Work out the finished part from the listing and answer in its coordinate system (mm). Face numbers are marked on the shaded views. A direction names the side the tool comes from. Give positions to 0.01 mm unless a question says otherwise; leave off trailing zeros. Loops run counter-clockwise (first coordinate to the right, second up) from the corner with the lowest first, then second, coordinate; pieces in that order, holes last.
```python
from build123d import *

# Parameters (mm, degrees)
EXTRUDE_1_DEPTH     = 18
HOLE_WIZARD_M6_1_D  = 5
SKETCH_6_R          = 3
CUT_EXTRUDE_1_DEPTH = 259.015029546
SKETCH_7_R          = 11
SKETCH_7_R_2        = 1.25
CUT_EXTRUDE_2_DEPTH = 259.015029546


with BuildPart() as part:
    # 草图1 → 凸台-拉伸1 (new body)
    with BuildSketch(Plane.XY):
        Polygon((0, 0), (80, 0), (80, 60), (22.986425339, 129.63800905), (22.986425339, 244.63800905), (-47.013574661, 244.63800905), (-47.013574661, 104.63800905), (0, 47.214285714), align=None)
    extrude(amount=EXTRUDE_1_DEPTH)

    # M6 螺纹孔1 (through all)
    with Locations(Plane.XY.offset(18)):
        with Locations((-40.013574661, 114.63800905), (-22.013574661, 114.63800905), (-40.013574661, 234.63800905), (-22.013574661, 234.63800905), (-42.013574661, 174.63800905)):
            Hole(HOLE_WIZARD_M6_1_D / 2)

    # 草图6 → 切除-拉伸1 (cut, through all)
    with BuildSketch(Plane.XY.offset(18)):
        with Locations((15, 20)):
            Circle(SKETCH_6_R)
        with Locations((65, 20)):
            Circle(SKETCH_6_R)
        with Locations((40, 20)):
            Circle(SKETCH_6_R)
    extrude(amount=-CUT_EXTRUDE_1_DEPTH, mode=Mode.SUBTRACT)

    # 草图7 → 切除-拉伸2 (cut, through all)
    with BuildSketch(Plane.XY.offset(18)):
        with Locations((-12.013574661, 174.63800905)):
            Circle(SKETCH_7_R)
        with Locations((-27.513574661, 190.13800905)):
            Circle(SKETCH_7_R_2)
        with Locations(Location((3.486425339, 190.13800905, 0), (0, 0, 180))):
            Circle(SKETCH_7_R_2)
        with Locations((3.486425339, 159.13800905)):
            Circle(SKETCH_7_R_2)
        with Locations(Location((-27.513574661, 159.13800905, 0), (0, 0, 180))):
            Circle(SKETCH_7_R_2)
    extrude(amount=-CUT_EXTRUDE_2_DEPTH, mode=Mode.SUBTRACT)


solid = part.part
```
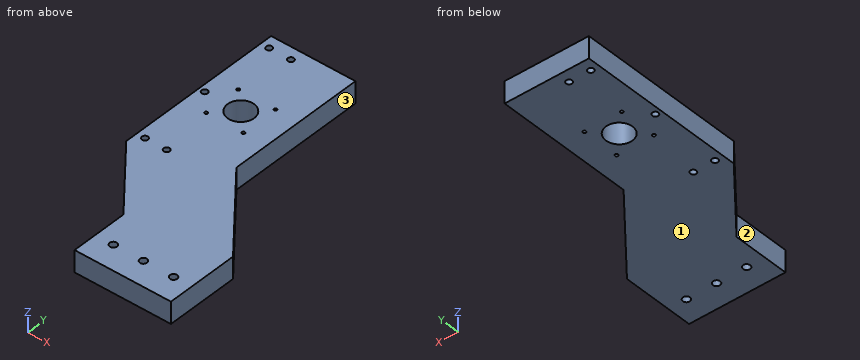
Q1. Section A-A on y = 20 is taken. Give the vertices of the cut face in (x, z), plus the area to 3 significant figures.
Q2. Which of the six approach directions +Z, -Z, +X, -X, +Y, -Y give full straight-line access (tool end or side, diameter ignored) to the marked faces 1, 2 and 3?
Q3. Given pin 1 (8 mm diameter, centred on x = -40.01, y = 234.64, fed in from -Z); pin 2 (5 mm diameter, centred on x = 33.5, z = 7, fed in from +Y); pin 3 (10 mm diameter, centred on y = 35, z = 3.5, fed in from -X); pin 4 (6 mm diameter, centred on x = -23, z = 7, fed in from -Y), each flat-ended and moving along its own axis, determine where each tip first touches the part or whether it passes through.
Q4. Consider line 1 along Y through (x, z) = (15, 14.75); line 2 along Y through (x, z) = (4.5, 16.75); line 3 along X through (y, z) = (22.5, 1.5). Determine where each line is inside the solid, lowest interval first.
Q5. Section D-D on x = 65 is taken. Give the vertices of the cut face in (y, z), plus the area to 3 significant figures.
Q6. Section C-C on z = 8.75 is taken. State how many separate pieces and enclosed holes the cut face has, plus the area to 3 significant figures.
Q7. Section B-B on x = 15 is taken. Give the vertices of the cut face in (y, z).
Check result:
1. outline: (0, 0) - (12, 0) - (12, 18) - (0, 18) - close; (18, 0) - (37, 0) - (37, 18) - (18, 18) - close; (43, 0) - (62, 0) - (62, 18) - (43, 18) - close; (68, 0) - (80, 0) - (80, 18) - (68, 18) - close
1. area: 1,120 mm2
2. face 1: -Z, +X, -X, +Y, -Y
2. face 2: +Z, -Z, -X, -Y
2. face 3: +Z, -Z, +X, +Y
3. pin 1: stops at z = 0
3. pin 2: stops at y = 119.85
3. pin 3: stops at x = 0
3. pin 4: stops at y = 71.64
4. line 1: y = 0 to 17, 23 to 244.64
4. line 2: y = 0 to 158.41, 159.87 to 189.41, 190.87 to 244.64
4. line 3: x = 0 to 13.34, 16.66 to 38.34, 41.66 to 63.34, 66.66 to 80
5. outline: (0, 0) - (17, 0) - (17, 18) - (0, 18) - close; (23, 0) - (78.32, 0) - (78.32, 18) - (23, 18) - close
5. area: 1,300 mm2
6. separate pieces: 1
6. enclosed holes: 13
6. area: 18,400 mm2
7. outline: (0, 0) - (17, 0) - (17, 18) - (0, 18) - close; (23, 0) - (244.64, 0) - (244.64, 18) - (23, 18) - close
